Work out the finished part from the listing and answer in its coordinate system (mm). A direction names the side the tool comes from. Give positions to 0.01 mm unless a question says otherwise; leave off trailing zeros. Loops run counter-clockwise (first coordinate to the right, second up) from the corner with the lowest first, then second, coordinate; pieces in that order, holes last. Notation, with made-up numbers: (24.5, 70) -> (80.5, 70) arc R31 cw to (80.5, 108) -> close; hole circle Ø3 at (60.25, 73). An arc over 180 degrees is marked (long way). Answer as CSV lines item,"result". Start each with the question number.
1. Find the intervals of material crossed by line 1 along Z through (x, y) = (-4.75, 24); line 2 along Z through (x, y) = (8.75, 24.5); line 3 along Z through (x, y) = (1.5, 0), in increasing order.
2. Find section D-D, the plane y = -15. Give the vertices of the cut face in (x, z), and give its area (3 significant figures).
3. A tool of negligible diameter and unlimited length cuts with its end or side. For faces 1 (the face through (1.15, 19.7, -7.17)), 2 (the face through (1.148, -19.704, 42.97)), 3 (the face through (1.1, 13.8, -6.6)), from which of +Z, -Z, +X, -X, +Y, -Y can it reach the whole face along a straight path? Write none if from no direction.
4. Find section C-C, the plane z = 37. Give the vertices of the cut face in (x, y).
5. Flat-ended cylindrical pins translate along their axes: pin 1 Ø10 at (x, z) = (-3.5, 11) entering from -Y; pin 2 Ø24 at (y, z) = (-12, 21.5) entering from +X; pin 3 Ø6 at (x, y) = (-0.5, -16) entering from +Z; pin 4 Ø23 at (y, z) = (0, 17.9) entering from -X. Find the tip coordinate at first contact, or state that the pin passes through.
6. Find section A-A, the plane y = 0. Give the vertices of the cut face in (x, z).
7. Determine the mould class of faces 4 (the face through (1.148, 31.564, 22.427)), 5 (the face through (1.148, -24.504, 4.112)), 6 (the face through (12.422, -23.5, 23.2)), 7 (the face through (0.83, 25, 43.07)) for opening direction Z: +Z half, -Z half, draft (parallel to the pull), parting line (faces both ways), or undercut.
8. Find section B-B, the plane z = -12. Give the vertices of the cut face in (x, y), and give its area (3 significant figures).
from build123d import *

# Parameters (mm, degrees)
F0_W     = 13.0011960864
F0_H     = 11.2356059253
F3_DEPTH = 35.5538306758
F4_COUNT = 12


with BuildPart() as f1:
    # F0 (on Front) → F1 (revolve)
    with BuildSketch(Plane.XZ):
        Polygon((12.4220475554, 53.374812007), (-10.4466825724, 53.374812007), (-10.4466825724, 41.814442724), (-5.5474191904, 41.814442724), (7.453776896, 41.814442724), (12.4220475554, 41.814442724), align=None)
        with Locations((0.9531788528, 36.1966397613)):
            Rectangle(F0_W, F0_H)
    revolve(axis=Axis((1.9577341154, 0, 17.8986564279), (1, 0, 0)))

    # F2 (on Right) → F3 (cut, symmetric)
    with BuildSketch(Plane.YZ):
        Polygon((6.6623128951, 55.3299412131), (-6.9674830884, 54.4798821211), (-2.8427802026, 45.9955856204), (3.5579316318, 46.0315644741), align=None)
    f3 = extrude(amount=F3_DEPTH, both=True, mode=Mode.SUBTRACT)

    # F4: F3 ×12 about axis
    f4_axis = Axis((12.4220475554, 0, 17.8986564279), (1, 0, 0))
    for i in range(1, F4_COUNT):
        add(f3.rotate(f4_axis, i * 360 / F4_COUNT), mode=Mode.SUBTRACT)


solid = f1.part
Resolved:
1,line 1,"z = -8.23 to -0.85, 3.23 to 32.55, 36.02 to 44.02"
1,line 2,"z = -7.76 to -1.41, 4.11 to 31.69, 36.76 to 43.56"
1,line 3,"z = -10.21 to 5.22, 30.58 to 46.01"
2,outline,"(-10.45, -5.91) -> (12.42, -5.91) -> (12.42, -0.73) -> (7.45, -0.73) -> (7.45, 36.53) -> (12.42, 36.53) -> (12.42, 41.69) -> (-10.45, 41.69) -> (-10.45, 36.53) -> (-5.55, 36.53) -> (-5.55, -0.73) -> (-10.45, -0.73) -> close"
2,area,"721 mm^2"
3,face 1,"-Z, +X, -X"
3,face 2,"+Z, +X, -X"
3,face 3,"+X, -X"
4,outline,"(-10.45, -24.32) -> (12.42, -24.32) -> (12.42, -14.39) -> (7.45, -14.39) -> (7.45, 14.39) -> (12.42, 14.39) -> (12.42, 24.66) -> (-10.45, 24.66) -> (-10.45, 14.39) -> (-5.55, 14.39) -> (-5.55, -14.39) -> (-10.45, -14.39) -> close"
5,pin 1,"stops at y = -34.94"
5,pin 2,"stops at x = 12.42"
5,pin 3,"stops at z = 42.86"
5,pin 4,"passes through"
6,outline,"(-10.45, -10.21) -> (12.42, -10.21) -> (12.42, -6.02) -> (7.45, -6.02) -> (7.45, 5.22) -> (-5.55, 5.22) -> (-5.55, -6.02) -> (-10.45, -6.02) -> close; (-10.45, 41.81) -> (-5.55, 41.81) -> (-5.55, 30.58) -> (7.45, 30.58) -> (7.45, 41.81) -> (12.42, 41.81) -> (12.42, 46.01) -> (-10.45, 46.01) -> close"
7,face 4,"undercut"
7,face 5,"undercut"
7,face 6,"draft"
7,face 7,"+Z half"
8,outline,"(-10.45, -11.88) -> (12.42, -11.88) -> (12.42, -4.15) -> (-10.45, -4.15) -> close; (-10.45, 3.72) -> (12.42, 3.72) -> (12.42, 11.75) -> (-10.45, 11.75) -> close"
8,area,"361 mm^2"
